Geometry: final body of the model. Coordinates: model frame, mm. A direction names the side the tool comes from. Coordinates: 2 decimals unless noted, no trailing zeros. Order: outer loops, then holes, each group sorted by start corner. A loop starts at its lowest first (then second) coordinate and runs counter-clockwise, first axis right, second up. Notation, with made-up numbers: (41, -7.5) - (88, -7.5) arc R11 ccw to (88, -3.5) - close; hole circle Ø2 at (-11, 24). An arc over 180 degrees is marked (long way). Use a Markdown table: item, result. Add a question column.
```python
from build123d import *

# Parameters (mm, degrees)
SKETCH2_W                    = 33.7
SKETCH2_H                    = 50
BOSS_EXTRUDE1_DEPTH          = 2
BOSS_EXTRUDE2_DEPTH          = 12.7
CUT_EXTRUDE1_REACH           = 45.84
SKETCH4_R                    = 2
SKETCH5_R                    = 11.5
SKETCH5_R_2                  = 5.5
BOSS_EXTRUDE3_DEPTH          = 4.1
CUT_EXTRUDE_THIN1_DEPTH      = 34.541206001
CUT_EXTRUDE_THIN1_DEPTH_BACK = 8.2
CUT_EXTRUDE2_REACH           = 54.433
SKETCH7_R                    = 2


with BuildPart() as part:
    # Sketch2 → Boss-Extrude1 (new body)
    with BuildSketch(Plane(origin=(0, 0, 0), x_dir=(1, 0, 0), z_dir=(0, 1, 0))):
        Rectangle(SKETCH2_W, SKETCH2_H)
    extrude(amount=BOSS_EXTRUDE1_DEPTH)

    # Sketch3 → Boss-Extrude2 (add)
    with BuildSketch(Plane.XZ):
        Polygon((14.85, 25), (14.85, -23), (-16.85, -23), (-16.85, -25), (16.85, -25), (16.85, 25), align=None)
    extrude(amount=BOSS_EXTRUDE2_DEPTH)

    # Sketch4 → Cut-Extrude1 (cut, up to next)
    with BuildSketch(Plane(origin=(16.85, 0, 0), x_dir=(0, 0, -1), z_dir=(1, 0, 0)), mode=Mode.PRIVATE) as cut_extrude1_sk1:
        with Locations((12.5, -3.5)):
            Circle(SKETCH4_R)
    cut_extrude1_tool1 = extrude(cut_extrude1_sk1.sketch, amount=-CUT_EXTRUDE1_REACH, mode=Mode.PRIVATE) & part.part
    # Sketch4 → Cut-Extrude1 (cut, up to next)
    with BuildSketch(Plane(origin=(16.85, 0, 0), x_dir=(0, 0, -1), z_dir=(1, 0, 0)), mode=Mode.PRIVATE) as cut_extrude1_sk2:
        with Locations((-12.5, -3.5)):
            Circle(SKETCH4_R)
    cut_extrude1_tool2 = extrude(cut_extrude1_sk2.sketch, amount=-CUT_EXTRUDE1_REACH, mode=Mode.PRIVATE) & part.part
    add(cut_extrude1_tool1.solids().sort_by_distance((16.85, -3.5, -12.5))[0], mode=Mode.SUBTRACT)
    add(cut_extrude1_tool2.solids().sort_by_distance((16.85, -3.5, 12.5))[0], mode=Mode.SUBTRACT)

    # Sketch5 → Boss-Extrude3 (add)
    with BuildSketch(Plane.XZ):
        with Locations(Location((-4, 0, 0), (0, 0, 90))):
            Circle(SKETCH5_R)
        with Locations(Location((-4, 0, 0), (0, 0, 270))):
            Circle(SKETCH5_R_2, mode=Mode.SUBTRACT)
    extrude(amount=BOSS_EXTRUDE3_DEPTH)

    # Sketch6 → Cut-Extrude-Thin1 (cut, two sides: drawn at the far end of the back side and taken through both)
    with BuildSketch(Plane(origin=(0, 2, 0), x_dir=(1, 0, 0), z_dir=(0, 1, 0)).offset(-CUT_EXTRUDE_THIN1_DEPTH_BACK)):
        with BuildLine():
            ThreePointArc((-16.85, 0), (-15.057855322, -6.545711243), (-10.181309623, -11.265607456))
            Line((-10.181309623, -11.265607456), (14.85, -25))
            Line((14.85, -25), (5.229284634, -42.534019386))
            Line((5.229284634, -42.534019386), (-19.802024989, -28.799626842))
            ThreePointArc((-19.802024989, -28.799626842), (-32.268525084, -16.733588663), (-36.85, 0))
            Line((-36.85, 0), (-16.85, 0))
        make_face()
    extrude(amount=CUT_EXTRUDE_THIN1_DEPTH + CUT_EXTRUDE_THIN1_DEPTH_BACK, mode=Mode.SUBTRACT)

    # Sketch7 → Cut-Extrude2 (cut, up to next)
    with BuildSketch(Plane.XY.offset(-23), mode=Mode.PRIVATE) as cut_extrude2_sk1:
        with Locations((-9.85, -6.35)):
            Circle(SKETCH7_R)
    cut_extrude2_tool1 = extrude(cut_extrude2_sk1.sketch, amount=-CUT_EXTRUDE2_REACH, mode=Mode.PRIVATE) & part.part
    # Sketch7 → Cut-Extrude2 (cut, up to next)
    with BuildSketch(Plane.XY.offset(-23), mode=Mode.PRIVATE) as cut_extrude2_sk2:
        with Locations((7.85, -6.35)):
            Circle(SKETCH7_R)
    cut_extrude2_tool2 = extrude(cut_extrude2_sk2.sketch, amount=-CUT_EXTRUDE2_REACH, mode=Mode.PRIVATE) & part.part
    add(cut_extrude2_tool1.solids().sort_by_distance((-9.85, -6.35, -23))[0], mode=Mode.SUBTRACT)
    add(cut_extrude2_tool2.solids().sort_by_distance((7.85, -6.35, -23))[0], mode=Mode.SUBTRACT)


solid = part.part
```
1) Section A-A (y = -3.5). Return loops of the section in (x, z), then the cut area to 3 significant figures.
2) Section B-B (z = 12.5). Return loops of the section in (x, y), then the cut area to 3 significant figures.
3) Draft query along Z for faces 1 (the face through (2.159, 0.986, 18.037)), 2 (the face through (0, 2, -6)), 3 (the face through (15.9, -4.7, 14.1)), 4 (the face through (0, -5, -25)). Return one class per face: pulls with the +Z half, pulls with the -Z half, needs draft (parallel to the pull), parting line crosses it, or undercut.
4) Ray query, line 1 along Y through (x, z) = (15.3, 12.5); line 2 along Y through (x, z) = (-9.85, -24); line 3 along Y through (x, z) = (-15, -14). Return the intervals inside material, ascending.
5) Section D-D (y = -7.25). Return loops of the section in (x, z), then the cut area to 3 significant figures.
6) Set-up query: faces 5 (the face through (-4, 0, 0)), 6 (the face through (-1, -6, -23)), 7 (the face through (14.85, -6, 1)). Return all of +Z, -Z, +X, -X, +Y, -Y with unobstructed straight access to the full face (end or side cutting, diameter ignored); none if empty.
7) Pin query (flat end, axial travel): pin 1 (3 mm diameter, centred on x = -9.85, y = -6.35, fed in from -Z); pin 2 (2 mm diameter, centred on x = 9, z = 1.5, fed in from -Y); pin 3 (7 mm diameter, centred on x = -5.5, z = -3, fed in from -Y); pin 4 (8 mm diameter, centred on y = -0.5, z = 20, fed in from -X). Return the tip coordinate at first contact, or that it passes through.
8) Section C-C (x = 7). Return loops of the section in (y, z), then the cut area to 3 significant figures.
Values follow:
| question | item | result |
|---|---|---|
| 1 | outline | (-16.85, -25) - (16.85, -25) - (16.85, -14.5) - (14.85, -14.5) - (14.85, -23) - (-16.85, -23) - close; circle Ø23 at (-4, 0); (14.85, -10.5) - (16.85, -10.5) - (16.85, 10.5) - (14.85, 10.5) - close; (14.85, 14.5) - (16.85, 14.5) - (16.85, 25) - (14.85, 25) - close; hole circle Ø11 at (-4, 0) |
| 1 | area | 468 mm² |
| 2 | outline | (-7.93, 0) - (14.85, 0) - (14.85, -1.5) - (16.85, -1.5) - (16.85, 2) - (-7.93, 2) - close; (14.85, -12.7) - (16.85, -12.7) - (16.85, -5.5) - (14.85, -5.5) - close |
| 2 | area | 67.0 mm² |
| 3 | face 1 | pulls with the +Z half |
| 3 | face 2 | needs draft |
| 3 | face 3 | undercut |
| 3 | face 4 | pulls with the -Z half |
| 4 | line 1 | y = -12.7 to -5.5, -1.5 to 2 |
| 4 | line 2 | y = -12.7 to -8.35, -4.35 to 2 |
| 4 | line 3 | y = 0 to 2 |
| 5 | outline | (-16.85, -25) - (-11.64, -25) - (-11.64, -23) - (-16.85, -23) - close; (-8.06, -25) - (6.06, -25) - (6.06, -23) - (-8.06, -23) - close; (9.64, -25) - (16.85, -25) - (16.85, 25) - (14.85, 25) - (14.85, -23) - (9.64, -23) - close |
| 5 | area | 149 mm² |
| 6 | face 5 | -Y |
| 6 | face 6 | -X, -Y |
| 6 | face 7 | +Z, -Y |
| 7 | pin 1 | passes through |
| 7 | pin 2 | stops at y = 0 |
| 7 | pin 3 | stops at y = -4.1 |
| 7 | pin 4 | stops at x = -1.5 |
| 8 | outline | (-12.7, -25) - (-8.16, -25) - (-8.16, -23) - (-12.7, -23) - close; (-4.54, -25) - (2, -25) - (2, 20.69) - (0, 20.69) - (0, 3.35) - (-4.1, 3.35) - (-4.1, -3.35) - (0, -3.35) - (0, -23) - (-4.54, -23) - close |
| 8 | area | 137 mm² |
